The model under review builds one solid part; all positions refer to its coordinate system, in mm. A direction names the side the tool comes from. Coordinates: 2 decimals unless noted, no trailing zeros. Write each loop counter-clockwise with the first axis right and the second up, starting at its lowest first coordinate (ties: lowest second). Pieces come first, ordered by that corner, then holes.
1) For P1, Ø4.5, axis at y = 7.5, z = 33, coming from the -X side; P2, Ø1.3, axis at x = -3.5, y = 7, coming from the -Z side; P3, Ø1.3, axis at y = 6, z = 30.5, coming from the +X side, all flat-tipped, find the tip position at first contact; note any pin that passes through.
2) Add section C-C, the plane z = -10. State the section outline as (x, y) points.
3) Add section D-D, the plane x = 13.5. State the section outline as (y, z) points.
4) Machinability: for faces 1 (the flat face through (0, 7, 22.485)), 2 (the flat face through (-8.467, 7, 32)), 3 (the flat face through (8.467, 7, 32)), which of the approach directions +Z, -Z, +X, -X, +Y, -Y give a long, thin tool a straight path to every point of the face, cutting with its end or side? Answer none if there is none.
5) For line 1 (Y direction, x = -3, z = -27); line 2 (Z direction, x = -1, y = 5); line 3 (X direction, y = 8, z = 36), list the stretches that pass through material, from the lowest coordinate up.
6) Add section B-B, the plane x = -4. State the section outline as (y, z) points.
7) Add section A-A, the plane z = 32. State the section outline as (x, y) points.
Autodesk Inventor part; units mm, degrees
ref_plane "YZ Plane" through (0, 0, 0) normal (1, 0, 0) x (0, 1, 0)
ref_plane "XZ Plane" through (0, 0, 0) normal (0, 1, 0) x (-1, 0, 0)
ref_plane "XY Plane" through (0, 0, 0) normal (0, 0, 1) x (1, 0, 0)
sketch "Sketch1" plane through (0, 0, 0) normal (0, 1, 0) x (-1, 0, 0)
  line L0 (-27.6479, 41.5354) -> (27.6479, 41.5354)
  line L1 (27.6479, 41.5354) -> (27.6479, -41.5354)
  line L2 (27.6479, -41.5354) -> (-27.6479, -41.5353)
  line L3 (-27.6479, -41.5353) -> (-27.6479, 41.5354)
  line L4 (-27.6479, 41.5354) -> (27.6479, -41.5354) construction
  line L5 (27.6479, 41.5354) -> (-27.6479, -41.5353) construction
  point P0 (0, 0)
  dimension "BreadboardWidth" = 55.2958
  dimension "BreadboardLength" = 83.0707
extrude "Breadbord" add sketch "Sketch1" along normal mid plane 9.398
sketch "Sketch2" plane through (0, 4.699, 0) normal (0, 1, 0) x (1, 0, 0)
  line L0 (8.4667, -41.5354) -> (-8.4667, -41.5354)
  line L1 (-8.4667, -41.5354) -> (-8.4667, -22.4854)
  line L2 (-8.4667, -22.4854) -> (8.4667, -22.4854)
  line L3 (8.4667, -22.4854) -> (8.4667, -41.5354)
  line L4 (8.4667, -41.5354) -> (-8.4667, -22.4854) construction
  line L5 (-8.4667, -41.5354) -> (8.4667, -22.4854) construction
  line L6 (27.6479, 41.5353) -> (-27.6479, 41.5354)
  line L7 (-27.6479, -41.5354) -> (27.6479, -41.5354)
  point P0 (0, 0)
  point P1 (0, -32.0104)
  dimension "d4" = 16.9333
  dimension "d5" = 19.05
extrude "LIDAR Chip" add sketch "Sketch2" along normal blind 4.2672
properties part number "Breadboard"
Geometry results:
1. P1: stops at x = -8.47
1. P2: stops at z = 22.49
1. P3: stops at x = 8.47
2. outline: (-27.65, -4.7) - (27.65, -4.7) - (27.65, 4.7) - (-27.65, 4.7) - close
3. outline: (-4.7, -41.54) - (4.7, -41.54) - (4.7, 41.54) - (-4.7, 41.54) - close
4. face 1: -Z, +X, -X, +Y
4. face 2: +Z, -Z, -X, +Y
4. face 3: +Z, -Z, +X, +Y
5. line 1: y = -4.7 to 4.7
5. line 2: z = 22.49 to 41.54
5. line 3: x = -8.47 to 8.47
6. outline: (-4.7, -41.54) - (4.7, -41.54) - (4.7, 22.49) - (8.97, 22.49) - (8.97, 41.54) - (-4.7, 41.54) - close
7. outline: (-27.65, -4.7) - (27.65, -4.7) - (27.65, 4.7) - (8.47, 4.7) - (8.47, 8.97) - (-8.47, 8.97) - (-8.47, 4.7) - (-27.65, 4.7) - close
